Can you work these out from the model? Positions are in its coordinate system, mm. A direction names the side the tool comes from. Give positions to 0.01 mm unless a question says otherwise; leave off trailing zeros. Order: outer loops, then holes, each group sorted by start corner. A loop starts at its lowest first (then second) coordinate and runs counter-clockwise, first axis right, second up.
Item 1: Which directions (+Z, -Z, +X, -X, +Y, -Y) give clear straight access to the entire face, cutting with the end or side of a thin tool? Please do faces 4 (the flat face through (-1, 1, 0)), 5 (the flat face through (-1, 1, 6.35)).
Item 2: If we mould it in two halves opening along Y, with no side actions, what happens to faces 1 (the flat face through (85.09, 1, 78)), 2 (the cylindrical face through (87.372, -87.451, 78.519)), 3 (the flat face through (-88.9, 1, 76))? For each: +Y half, -Y half, draft (parallel to the pull), parting line (faces both ways), or undercut.
Item 3: I want a section at B-B, the plane y = 1.5. Write out the boundary of the cut face in (x, z).
Item 4: If I drill on line 1 along X through (y, z) = (-69, 77); line 2 along Z through (x, y) = (22.5, -4), over which ranges is the centre line in solid material (lowest first)?
Item 5: I want a section at A-A, the plane z = 101. Write out the boundary of the cut face in (x, y).
```python
from build123d import *

# Parameters (mm, degrees)
F1_DEPTH = 152.4
F2_DEPTH = 6.35
F4_R     = 5.08
F5_R     = 2.54


# Not quite as in the source:
# - ends of sketch curves that miss each other by under 0.0002 mm in the source are joined


with BuildPart() as f1:
    # F0 (on Top) → F1 (new body)
    with BuildSketch(Plane.XY):
        Polygon((88.9, 1.431e-07), (88.9, 88.9), (0, 88.9), (0, 85.09), (85.09, 85.09), (85.09, 1.431e-07), align=None)
        Polygon((0, 85.09), (0, 88.9000001431), (-88.9, 88.9), (-88.9, 1.431e-07), (-85.09, 1.431e-07), (-85.09, 85.09), align=None)
        Polygon((-85.09, 1.431e-07), (-88.9, 1.431e-07), (-88.9, -88.9), (0, -88.9), (0, -85.09), (-85.09, -85.09), align=None)
        Polygon((88.9, -88.9), (88.9, 1.431e-07), (85.09, 1.431e-07), (85.09, -85.09), (0, -85.09), (0, -88.8999998569), align=None)
    extrude(amount=F1_DEPTH)

    # F0 (on Top) → F2 (join)
    with BuildSketch(Plane.XY):
        Polygon((85.09, -85.09), (85.09, 1.431e-07), (57.15, 1.431e-07), (44.45, 1.431e-07), (31.75, 1.431e-07), (0, 1.431e-07), (0, -31.7499998569), (10.16, -26.6699998569), (10.16, -44.4499998569), (10.16, -62.2299998569), (0, -57.1499998569), (0, -85.09), align=None)
        Polygon((0, 57.1500001431), (0, 85.09), (-85.09, 85.09), (-85.09, 1.431e-07), (-57.15, 1.431e-07), (-44.45, 1.431e-07), (-31.75, 1.431e-07), (0, 1.431e-07), (0, 31.7500001431), (-10.16, 26.6700001431), (-10.16, 44.4500001431), (-10.16, 62.2300001431), align=None)
        Polygon((44.45, 1.431e-07), (57.15, 1.431e-07), (62.23, 10.1600001431), (44.45, 10.1600001431), align=None)
        Polygon((31.75, 1.431e-07), (44.45, 1.431e-07), (44.45, 10.1600001431), (26.67, 10.1600001431), align=None)
        Polygon((0, 31.7500001431), (0, 44.4500001431), (-10.16, 44.4500001431), (-10.16, 26.6700001431), align=None)
        Polygon((0, 44.4500001431), (0, 57.1500001431), (-10.16, 62.2300001431), (-10.16, 44.4500001431), align=None)
        Polygon((85.09, 85.09), (0, 85.09), (0, 57.1500001431), (0, 44.4500001431), (0, 31.7500001431), (0, 1.431e-07), (31.75, 1.431e-07), (26.67, 10.1600001431), (44.45, 10.1600001431), (62.23, 10.1600001431), (57.15, 1.431e-07), (85.09, 1.431e-07), align=None)
        Polygon((-57.15, 1.431e-07), (-85.09, 1.431e-07), (-85.09, -85.09), (0, -85.09), (0, -57.1499998569), (0, -44.4499998569), (0, -31.7499998569), (0, 1.431e-07), (-31.75, 1.431e-07), (-26.67, -10.1599998569), (-44.45, -10.1599998569), (-62.23, -10.1599998569), align=None)
        Polygon((0, -31.7499998569), (0, -44.4499998569), (10.16, -44.4499998569), (10.16, -26.6699998569), align=None)
        Polygon((0, -44.4499998569), (0, -57.1499998569), (10.16, -62.2299998569), (10.16, -44.4499998569), align=None)
        Polygon((-31.75, 1.431e-07), (-44.45, 1.431e-07), (-44.45, -10.1599998569), (-26.67, -10.1599998569), align=None)
        Polygon((-44.45, 1.431e-07), (-57.15, 1.431e-07), (-62.23, -10.1599998569), (-44.45, -10.1599998569), align=None)
    extrude(amount=F2_DEPTH)

    # F4
    f4_edges = [f1.edges().sort_by_distance(p)[0] for p in [
        (-88.9, 88.9, 76.2),
        (88.9, 88.9, 76.2),
        (88.9, -88.9, 76.2),
        (-88.9, -88.9, 76.2),
    ]]
    fillet(f4_edges, radius=F4_R)

    # F5
    f5_edges = [f1.edges().sort_by_distance(p)[0] for p in [
        (41.91, 88.9, 0),
        (87.412102, 87.412102, 0),
        (-41.91, 88.9, 0),
        (88.9, 0, 0),
        (-87.412102, 87.412102, 0),
        (87.412102, -87.412102, 0),
        (-88.9, 0, 0),
        (41.91, -88.9, 0),
        (-87.412102, -87.412102, 0),
        (-41.91, -88.9, 0),
    ]]
    fillet(f5_edges, radius=F5_R)


solid = f1.part
```
Results list:
1. face 4: -Z, +X, -X, +Y, -Y
1. face 5: +Z
2. face 1: undercut
2. face 2: -Y half
2. face 3: draft
3. outline: (-88.9, 2.54) arc R2.54 ccw to (-86.36, 0) - (86.36, 0) arc R2.54 ccw to (88.9, 2.54) - (88.9, 152.4) - (85.09, 152.4) - (85.09, 6.35) - (-85.09, 6.35) - (-85.09, 152.4) - (-88.9, 152.4) - close
4. line 1: x = -88.9 to -85.09, 85.09 to 88.9
4. line 2: z = 0 to 6.35
5. outline: (-88.9, -83.82) arc R5.08 ccw to (-83.82, -88.9) - (83.82, -88.9) arc R5.08 ccw to (88.9, -83.82) - (88.9, 83.82) arc R5.08 ccw to (83.82, 88.9) - (-83.82, 88.9) arc R5.08 ccw to (-88.9, 83.82) - close; hole (-85.09, -85.09) - (85.09, -85.09) - (85.09, 85.09) - (-85.09, 85.09) - close
